Part print with two shaded views. Sizes in mm from the minimum x, y, z corner. A direction names the side the tool comes from. Round coordinates to 2 decimals unless told otherwise and drop trailing zeros. Order: outer loops, then holes, each group sorted by start corner. A loop starts at its lowest first (then second) coordinate and runs counter-clockwise, first axis right, second up. Notation, with made-up numbers: (42.5, 21) -> (67.5, 21) arc R15 ccw to (67.5, 31) -> close; hole circle Ø11 at (-24, 48). An arc over 180 degrees is marked (long way). Answer as a JSON object with one key per item and string values.
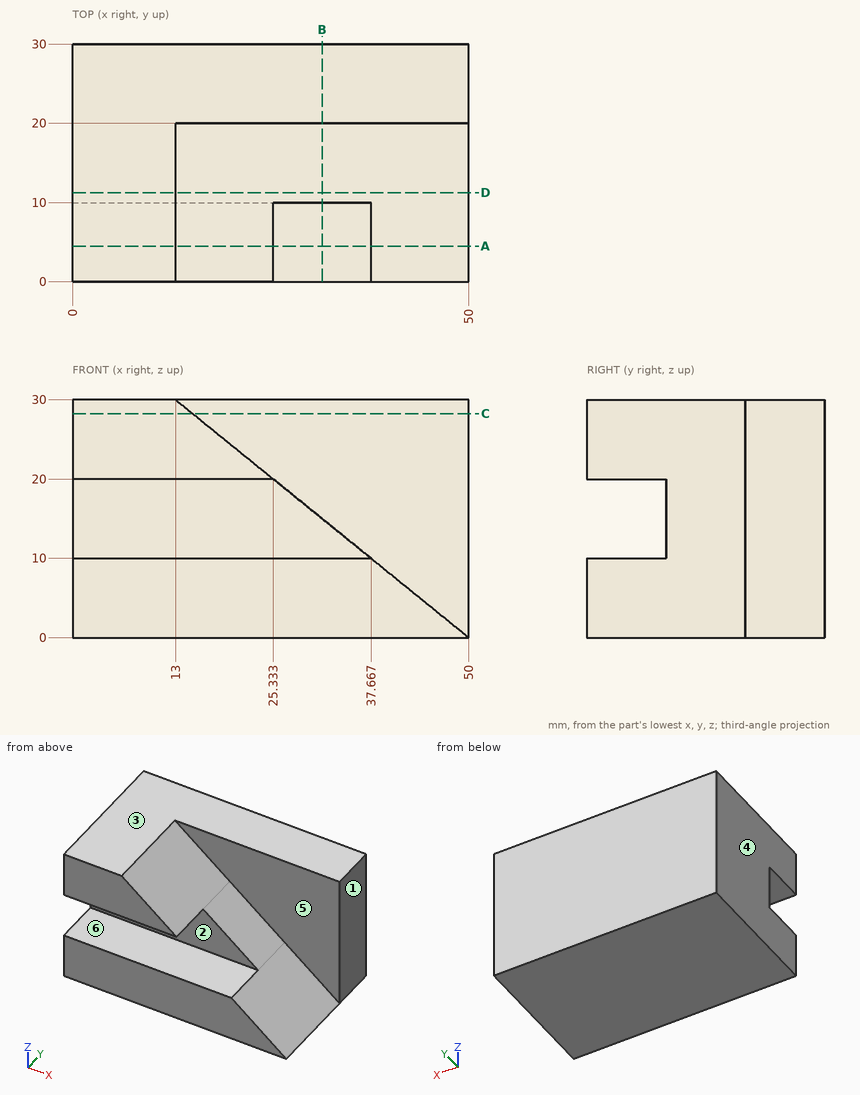
1) Flat gauge pins, fed straight in: pin 1 Ø2 at (y, z) = (24.5, 18) entering from -X; pin 2 Ø8 at (x, y) = (26, 8.5) entering from +Z; pin 3 Ø3 at (x, y) = (43, 9) entering from +Z; pin 4 Ø3 at (y, z) = (5.5, 6) entering from +X. Where does each tip first touch, or does it go through?
Checked values:
{"pin 1": "stops at x = 0", "pin 2": "stops at z = 22.7", "pin 3": "stops at z = 6.89", "pin 4": "stops at x = 44.45"}
2) Cut at B-B, the plane x = 31.5. Give the cut face in (y, z), plus the area to 3 significant figures.
Checked values:
{"outline": "(0, 0) -> (30, 0) -> (30, 30) -> (20, 30) -> (20, 15) -> (10, 15) -> (10, 10) -> (0, 10) -> close", "area": "550 mm²"}
3) Probe L1, parallel to Z at x = 25.5, y = 6; L2, parallel to Y at x = 37, z = 15; L3, parallel to Y at x = 14, z = 15. List the from-to ranges inside material, lowest first. Write a range as from..to.
Checked values:
{"L1": "z = 0..10", "L2": "y = 20..30", "L3": "y = 10..30"}
4) Cut at A-A, the plane y = 4.5. Give the cut face in (x, z).
Checked values:
{"outline": "(0, 0) -> (50, 0) -> (37.67, 10) -> (0, 10) -> close; (0, 20) -> (25.33, 20) -> (13, 30) -> (0, 30) -> close"}
5) Cut at C-C, the plane z = 28.25. Give the cut face in (x, y).
Checked values:
{"outline": "(0, 0) -> (15.16, 0) -> (15.16, 20) -> (50, 20) -> (50, 30) -> (0, 30) -> close"}
6) Pull direction Z, two halves, no side cores. Call the marked faces 1, 2 and 3: pulls with the +Z half, pulls with the -Z half, needs draft (parallel to the pull), parting line crosses it, or undercut.
Checked values:
{"face 1": "needs draft", "face 2": "undercut", "face 3": "pulls with the +Z half"}
7) Cut at D-D, the plane y = 11.25. Give the cut face in (x, z), plus the area to 3 significant figures.
Checked values:
{"outline": "(0, 0) -> (50, 0) -> (13, 30) -> (0, 30) -> close", "area": "945 mm²"}
8) Which spindle directions (+Z, -Z, +X, -X, +Y, -Y) get a long thin tool onto all of the face, cutting with end or side? Do the marked faces 4, 5 and 6. Say none if no direction does.
Checked values:
{"face 4": "+Z, -Z, -X, +Y, -Y", "face 5": "+Z, +X, -Y", "face 6": "+X, -X, -Y"}
